Can you work these out from the model? Positions are in its coordinate system, mm. Round coordinates to 2 decimals unless told otherwise and drop trailing zeros. Loops run counter-clockwise (first coordinate to the right, second up) from the corner with the lowest first, then second, coordinate; pieces in that order, holes last.
(1) I want a section at B-B on x = 0. Write out the boundary of the cut face in (y, z).
(2) I want a section at A-A on z = -6. Write out the boundary of the cut face in (x, y).
(3) Will these pins go through, and if not, where does the flat tip stop? pin 1 Ø1 at (y, z) = (-2.5, -5) entering from -X; pin 2 Ø2 at (x, y) = (21.5, -2) entering from -Z.
(4) If I drill on line 1 along Z through (x, y) = (-3, -0.55); line 2 along X through (y, z) = (-4, 4); line 3 along X through (y, z) = (-4.5, -7), over which ranges is the centre line in solid material (lowest first)?
(5) I want a section at C-C on x = 51. Write out the boundary of the cut face in (y, z), plus the area to 3 significant figures.
(6) I want a section at D-D on y = -4.9. Write out the boundary of the cut face in (x, z), plus the area to 3 significant figures.
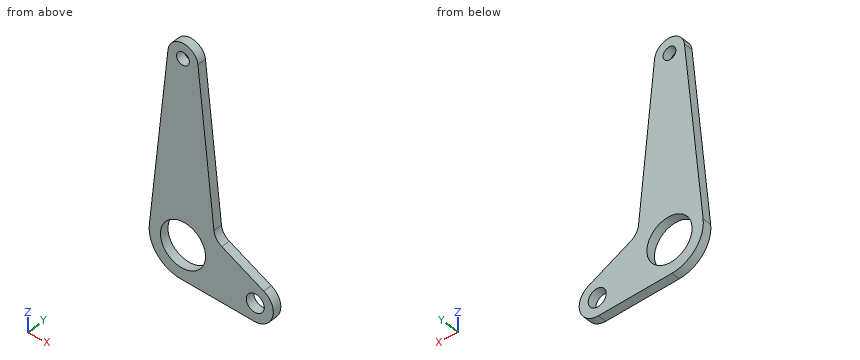
from build123d import *

# Parameters (mm, degrees)
F0_R     = 15
F0_R_2   = 6
F0_R_3   = 4.25
F1_DEPTH = 6


with BuildPart() as f1:
    # F0 (on Front) → F1 (new body)
    with BuildSketch(Plane.XZ):
        with BuildLine():
            Line((-9.945599, 121.041667), (-22.377597, 2.34375))
            ThreePointArc((-22.377597, 2.34375), (-17.217914, -14.484248), (-1.521587, -22.448492))
            Line((-1.521587, -22.448492), (47.251572, -25.754397))
            ThreePointArc((47.251572, -25.754397), (59.597932, -17.090538), (53.721232, -3.199554))
            Line((53.721232, -3.199554), (25.814877, 11.721405))
            ThreePointArc((25.814877, 11.721405), (22.232244, 14.959028), (20.584437, 19.497993))
            Line((20.584437, 19.497993), (9.945599, 121.041667))
            ThreePointArc((9.945599, 121.041667), (0, 130), (-9.945599, 121.041667))
        make_face()
        Circle(F0_R, mode=Mode.SUBTRACT)
        with Locations((48.063085, -13.781868)):
            Circle(F0_R_2, mode=Mode.SUBTRACT)
        with Locations((0, 120)):
            Circle(F0_R_3, mode=Mode.SUBTRACT)
    extrude(amount=F1_DEPTH)


solid = f1.part
Filled sheet:
1. outline: (-6, -22.55) - (0, -22.55) - (0, -15) - (-6, -15) - close; (-6, 15) - (0, 15) - (0, 115.75) - (-6, 115.75) - close; (-6, 124.25) - (0, 124.25) - (0, 130) - (-6, 130) - close
2. outline: (-21.69, -6) - (-13.75, -6) - (-13.75, 0) - (-21.69, 0) - close; (13.75, -6) - (57.2, -6) - (57.2, 0) - (13.75, 0) - close
3. pin 1: stops at x = -22.05
3. pin 2: stops at z = -24.08
4. line 1: z = -22.3 to -14.7, 14.7 to 116.99, 123.01 to 129.54
4. line 2: x = -22.2 to -14.46, 14.46 to 40.26
4. line 3: x = -21.38 to -13.27, 13.27 to 57.96
5. outline: (-6, -25.42) - (0, -25.42) - (0, -19.01) - (-6, -19.01) - close; (-6, -8.55) - (0, -8.55) - (0, -1.74) - (-6, -1.74) - close
5. area: 79.2 mm2
6. outline: (-22.38, 2.34) arc R22.5 ccw to (-1.52, -22.45) - (47.25, -25.75) arc R12 ccw to (53.72, -3.2) - (25.81, 11.72) arc R10 cw to (20.58, 19.5) - (9.95, 121.04) arc R10 ccw to (-9.95, 121.04) - close; hole circle Ø30 at (0, 0); hole circle Ø8.5 at (0, 120); hole circle Ø12 at (48.06, -13.78)
6. area: 5,170 mm2
